Geometry: see drawing. Coordinates: mm, zero at the bounding-box minimum. A direction names the side the tool comes from. Give positions to 0.01 mm unless a question says otherwise; leave off trailing zeros. Write each loop counter-clockwise with the first axis right and the second up, starting at its lowest first coordinate (ties: lowest second). Pieces come first, ordered by that corner, then holes. Notation, with made-up numbers: (-14.5, 63.5) - (38.5, 63.5) arc R14 ccw to (38.5, 68.5) - close; hole circle Ø1 at (56, -39). An arc over 180 degrees is marked (long way). Return JSON: item names as keys, results as strings.
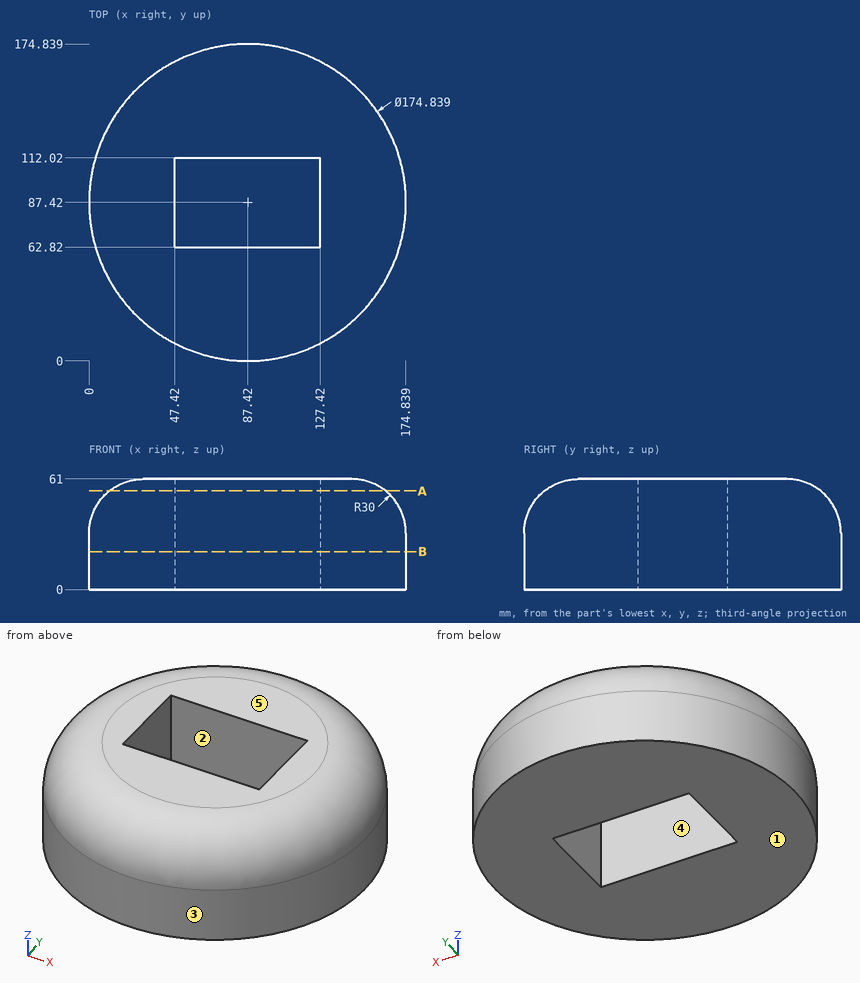
Q1. Section query A-A, the plane z = 54.5. Return the cut outline in (x, y) (1 decimal).
Answer key:
{"outline": "circle Ø152.1 at (87.4, 87.4); hole (47.4, 62.8) - (127.4, 62.8) - (127.4, 112) - (47.4, 112) - close"}
Q2. Material intervals for probe 1 along X at (y, z) = (88, 30); probe 2 along Y at (x, z) = (118, 50); probe 3 along Y at (x, z) = (48, 20), sorted ascending. Write a range as [from, to].
Answer key:
{"probe 1": "x = [0, 47.42], [127.42, 174.84]", "probe 2": "y = [12.81, 62.82], [112.02, 162.03]", "probe 3": "y = [9.39, 62.82], [112.02, 165.45]"}
Q3. Mould query, pull axis Y, two halves, no side actions, for the marked faces 3, 4 and 5. Classes: pulls with the +Y half, pulls with the -Y half, needs draft (parallel to the pull), parting line crosses it, or undercut.
Answer key:
{"face 3": "parting line crosses it", "face 4": "undercut", "face 5": "needs draft"}
Q4. Pin query (flat end, axial travel): P1, Ø5, axis at x = 144, z = 19.5, coming from the +Y side (1 decimal); P2, Ø1, axis at x = 29, y = 113.5, coming from the +Z side; P3, Ø4, axis at x = 148.5, z = 18.5, coming from the +Y side. Return the tip coordinate at first contact, or that it passes through.
Answer key:
{"P1": "stops at y = 156.1", "P2": "stops at z = 60.38", "P3": "stops at y = 151.85"}
Q5. Set-up query: the marked faces 1 and 2. Return all of +Z, -Z, +X, -X, +Y, -Y with unobstructed straight access to the full face (end or side cutting, diameter ignored); none if empty.
Answer key:
{"face 1": "-Z, +X, -X, +Y, -Y", "face 2": "+Z, -Z"}
Q6. Section query B-B, the plane z = 21. Return the cut outline in (x, y).
Answer key:
{"outline": "circle Ø174.84 at (87.42, 87.42); hole (47.42, 62.82) - (127.42, 62.82) - (127.42, 112.02) - (47.42, 112.02) - close"}
